Geometry: final body of the model. Coordinates: model frame, mm. A direction names the side the tool comes from. Round coordinates to 2 decimals unless told otherwise and drop trailing zeros. Write each loop counter-clockwise with the first axis right and the second up, starting at its lowest first coordinate (ties: lowest second). Pieces come first, ordered by that corner, then holes.
from build123d import *

# Parameters (mm, degrees)
F0_W     = 85.09
F0_H     = 95.25
F1_DEPTH = 19.05
F2_W     = 3.175
F2_H     = 101.6
F3_DEPTH = 6.35
F4_W     = 19.05
F4_H     = 6.35
F5_DEPTH = 85.091


with BuildPart() as f1:
    # F0 (on Top) → F1 (new body)
    with BuildSketch(Plane.XY):
        Rectangle(F0_W, F0_H)
    extrude(amount=F1_DEPTH)

    # F2 (on face) → F3 (cut)
    with BuildSketch(Plane.XY.offset(19.05)):
        with Locations((-31.75, 0)):
            Rectangle(F2_W, F2_H)
        with Locations((-19.05, 0)):
            Rectangle(F2_W, F2_H)
        with Locations((-6.35, 0)):
            Rectangle(F2_W, F2_H)
        with Locations((6.35, 0)):
            Rectangle(F2_W, F2_H)
        with Locations((19.05, 0)):
            Rectangle(F2_W, F2_H)
        with Locations((31.75, 0)):
            Rectangle(F2_W, F2_H)
    extrude(amount=-F3_DEPTH, mode=Mode.SUBTRACT)

    # F4 (on face) → F5 (cut, through all)
    with BuildSketch(Plane.YZ.offset(42.545)):
        with Locations((-38.1, 15.875)):
            Rectangle(F4_W, F4_H)
    extrude(amount=-F5_DEPTH, mode=Mode.SUBTRACT)


solid = f1.part
1) Section A-A on z = 15.5. Output: boundary loops of the cut face in (x, y) (1 decimal).
2) Section C-C on x = 34.5. Output: boundary loops of the cut face in (y, z) (3 decimals).
3) Line query: probe 1 along Y at (x, z) = (-38.5, 17) (3 decimals); probe 2 along Z at (x, y) = (20, -6). Output: solid intervals per line, ascending.
4) First-contact query: P1, Ø3, axis at x = -38.5, z = 15, coming from the -Y side (3 decimals). Flat tip, straight axial feed; report the tip coordinate or a pass-through.
5) Reachability of faces 1 (the flat face through (-7.938, 9, 16)), 2 (the flat face through (-13, 10, 19.05)), 3 (the flat face through (-25, -28.575, 16)) from +Z, -Z, +X, -X, +Y, -Y: full face, straight path, thin tool, end or side. Return the list, or none.
6) Section D-D on x = 19. Output: boundary loops of the cut face in (y, z) (3 decimals).
7) Draft query along X for faces 4 (the flat face through (-30.162, 9, 16)), 5 (the flat face through (-38, -28.575, 16)), 6 (the flat face through (42.545, -1, 9)). Return one class per face: pulls with the +X half, pulls with the -X half, needs draft (parallel to the pull), parting line crosses it, or undercut.
Filled in:
1. outline: (-42.5, -28.6) - (-33.3, -28.6) - (-33.3, 47.6) - (-42.5, 47.6) - close; (-30.2, -28.6) - (-20.6, -28.6) - (-20.6, 47.6) - (-30.2, 47.6) - close; (-17.5, -28.6) - (-7.9, -28.6) - (-7.9, 47.6) - (-17.5, 47.6) - close; (-4.8, -28.6) - (4.8, -28.6) - (4.8, 47.6) - (-4.8, 47.6) - close; (7.9, -28.6) - (17.5, -28.6) - (17.5, 47.6) - (7.9, 47.6) - close; (20.6, -28.6) - (30.2, -28.6) - (30.2, 47.6) - (20.6, 47.6) - close; (33.3, -28.6) - (42.5, -28.6) - (42.5, 47.6) - (33.3, 47.6) - close
2. outline: (-47.625, 0) - (47.625, 0) - (47.625, 19.05) - (-28.575, 19.05) - (-28.575, 12.7) - (-47.625, 12.7) - close
3. probe 1: y = -28.575 to 47.625
3. probe 2: z = 0 to 12.7
4. P1: stops at y = -28.575
5. face 1: +Z, +Y, -Y
5. face 2: +Z, +X, -X, +Y, -Y
5. face 3: +Z, +X, -X, -Y
6. outline: (-47.625, 0) - (47.625, 0) - (47.625, 12.7) - (-47.625, 12.7) - close
7. face 4: undercut
7. face 5: needs draft
7. face 6: pulls with the +X half
